Verification items for the finished model (mm, model axes). A direction names the side the tool comes from. Round coordinates to 2 decimals unless told otherwise and drop trailing zeros. Write each loop counter-clockwise with the first axis right and the second up, starting at its lowest first coordinate (ties: lowest second). Pieces come first, ordered by that corner, then holes. Notation, with made-up numbers: M -23,75.25 L -12,75.25 A34 cw -12,113.25 Z; hole C 14.25,71 d4. An arc over 180 degrees is marked long. One line per item, written item: value. Start each with the question number.
from build123d import *

# Parameters (mm, degrees)
SKETCH1_W           = 89.9
SKETCH1_H           = 29.8
BOSS_EXTRUDE1_DEPTH = 3
SKETCH8_R           = 1.5
SKETCH8_W           = 4
SKETCH8_H           = 10
CUT_EXTRUDE5_DEPTH  = 5
SKETCH12_W          = 5.5
SKETCH12_H          = 6.5
CUT_EXTRUDE8_DEPTH  = 10
SKETCH15_W          = 4
SKETCH15_H          = 29.8
BOSS_EXTRUDE2_DEPTH = 8.5
SKETCH16_W          = 4.7
SKETCH16_H          = 1.8
BOSS_EXTRUDE3_DEPTH = 4


with BuildPart() as part:
    # Sketch1 → Boss-Extrude1 (new body)
    with BuildSketch(Plane(origin=(0, 0, 0), x_dir=(1, 0, 0), z_dir=(0, 1, 0))):
        with Locations((44.95, 14.9)):
            Rectangle(SKETCH1_W, SKETCH1_H)
    extrude(amount=BOSS_EXTRUDE1_DEPTH)

    # Sketch8 → Cut-Extrude5 (cut)
    with BuildSketch(Plane(origin=(0, 0, 0), x_dir=(-1, 0, 0), z_dir=(0, -1, 0))):
        with Locations(Location((-87.9, 15, 0), (0, 0, 90))):
            Circle(SKETCH8_R)
        with Locations((-87.9, 5)):
            Rectangle(SKETCH8_W, SKETCH8_H)
        with Locations((-87.9, 24.8)):
            Rectangle(SKETCH8_W, SKETCH8_H)
    extrude(amount=-CUT_EXTRUDE5_DEPTH, mode=Mode.SUBTRACT)

    # Sketch12 → Cut-Extrude8 (cut)
    with BuildSketch(Plane.XZ):
        with Locations((79.15, -17.05)):
            Rectangle(SKETCH12_W, SKETCH12_H)
    extrude(amount=-CUT_EXTRUDE8_DEPTH, mode=Mode.SUBTRACT)

    # Sketch15 → Boss-Extrude2 (add)
    with BuildSketch(Plane(origin=(0, 3, 0), x_dir=(1, 0, 0), z_dir=(0, 1, 0))):
        with Locations((2, 14.9)):
            Rectangle(SKETCH15_W, SKETCH15_H)
    extrude(amount=BOSS_EXTRUDE2_DEPTH)

    # Sketch16 → Boss-Extrude3 (add)
    with BuildSketch(Plane(origin=(4, 0, 0), x_dir=(0, 0, -1), z_dir=(1, 0, 0))):
        with Locations((6.65, 9.4)):
            Rectangle(SKETCH16_W, SKETCH16_H)
        with Locations((23.15, 9.4)):
            Rectangle(SKETCH16_W, SKETCH16_H)
    extrude(amount=BOSS_EXTRUDE3_DEPTH)


solid = part.part
1) Access from +Z, -Z, +X, -X, +Y, -Y to the whole of each face (thin tool, end or side, straight path). Record for faces 4 (the flat face through (8, 9, -23)), 5 (the flat face through (6, 9, -20.8)), 6 (the flat face through (88, 1, -10)).
2) Mould release check, pull along Y, two halves, no side actions. Record for faces 1 (the flat face through (79, 1, -20.3)), 2 (the flat face through (44, 0, -15)), 3 (the flat face through (6, 8.5, -23)): pulls with the +Y half, pulls with the -Y half, needs draft (parallel to the pull), parting line crosses it, or undercut.
3) Cross-section at C-C (x = 87.9). Record the boundary of the cut face in (y, z).
4) Cross-section at B-B (y = 1.5). Record the boundary of the cut face in (x, z), then the cut area to 3 significant figures.
5) Thickness scan on line 1 (X direction, y = 1.5, z = -15); line 2 (Z direction, x = 87.9, y = 1.1); line 3 (Z direction, x = 5.5, y = 10). Record the ranges inside material, lowest first.
6) Cross-section at D-D (z = -22.25). Record the boundary of the cut face in (x, y).
7) Gauge pin test, flat ends, axial feed: pin 1 Ø5 at (x, y) = (20.5, 7) entering from +Z (3 decimals); pin 2 Ø1.5 at (x, y) = (88.5, 1.5) entering from +Z; pin 3 Ø2.5 at (y, z) = (6, -20) entering from +X; pin 4 Ø1.4 at (x, y) = (6.5, 10) entering from -Z. Record the tip position at first contact, or that the pin passes through.
8) Cross-section at A-A (z = -15). Record the boundary of the cut face in (x, y).
Results below:
1. face 4: +Z, -Z, +X, +Y
1. face 5: +X, +Y
1. face 6: +Z, +X, +Y, -Y
2. face 1: needs draft
2. face 2: pulls with the -Y half
2. face 3: undercut
3. outline: M 0,-19.8 L 3,-19.8 L 3,-16.5 L 0,-16.5 Z; M 0,-13.5 L 3,-13.5 L 3,-10 L 0,-10 Z
4. outline: M 0,-29.8 L 85.9,-29.8 L 85.9,-19.8 L 89.9,-19.8 L 89.9,-10 L 85.9,-10 L 85.9,0 L 0,0 Z; hole M 76.4,-20.3 L 81.9,-20.3 L 81.9,-13.8 L 76.4,-13.8 Z; hole C 87.9,-15 d3
4. area: 2,560 mm²
5. line 1: x = 0 to 76.4, 81.9 to 86.4, 89.4 to 89.9
5. line 2: z = -19.8 to -16.5, -13.5 to -10
5. line 3: z = -25.5 to -20.8, -9 to -4.3
6. outline: M 0,0 L 85.9,0 L 85.9,3 L 4,3 L 4,8.5 L 8,8.5 L 8,10.3 L 4,10.3 L 4,11.5 L 0,11.5 Z
7. pin 1: passes through
7. pin 2: stops at z = -10
7. pin 3: stops at x = 4
7. pin 4: stops at z = -25.5
8. outline: M 0,0 L 76.4,0 L 76.4,3 L 4,3 L 4,11.5 L 0,11.5 Z; M 81.9,0 L 86.4,0 L 86.4,3 L 81.9,3 Z; M 89.4,0 L 89.9,0 L 89.9,3 L 89.4,3 Z
